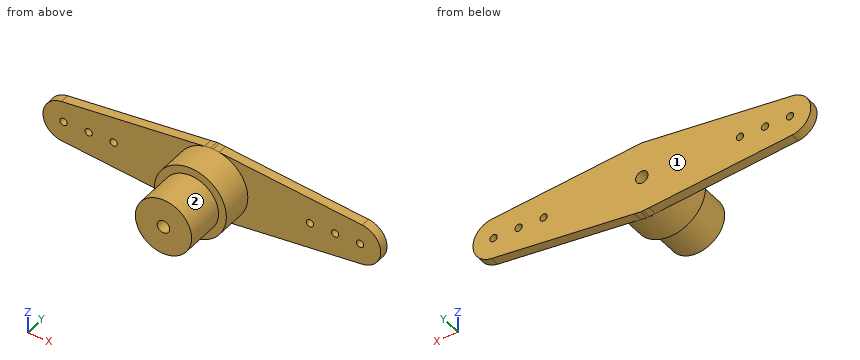
```python
from build123d import *

# Parameters (mm, degrees)
SKETCH1_R           = 2.875
BOSS_EXTRUDE1_DEPTH = 2.55
SKETCH1_4_R         = 0.291434634
BOSS_EXTRUDE2_DEPTH = 0.75
SKETCH2_R           = 2.25
BOSS_EXTRUDE3_DEPTH = 3.2
SKETCH3_R           = 0.5
CUT_EXTRUDE1_DEPTH  = 7.5
FILLET1_R           = 1


with BuildPart() as part:
    # Sketch1 → Boss-Extrude1 (new body)
    with BuildSketch(Plane(origin=(0, 0, 0), x_dir=(1, 0, 0), z_dir=(0, 1, 0))):
        Circle(SKETCH1_R)
    extrude(amount=-BOSS_EXTRUDE1_DEPTH)

    # Sketch1_4 → Boss-Extrude2 (add)
    with BuildSketch(Plane(origin=(0, 0, 0), x_dir=(1, 0, 0), z_dir=(0, 1, 0))):
        with BuildLine():
            Line((-0.584049273, 2.815050878), (-12.018477316, 1.641376067))
            ThreePointArc((-12.018477316, 1.641376067), (-13.5, 0), (-12.018477316, -1.641376067))
            Line((-12.018477316, -1.641376067), (-0.584049273, -2.815050878))
            ThreePointArc((-0.584049273, -2.815050878), (-2.875, 0), (-0.584049273, 2.815050878))
        make_face()
        with Locations((-11.85, 0)):
            Circle(SKETCH1_4_R, mode=Mode.SUBTRACT)
        with Locations((-9.85, 0)):
            Circle(SKETCH1_4_R, mode=Mode.SUBTRACT)
        with Locations((-7.85, 0)):
            Circle(SKETCH1_4_R, mode=Mode.SUBTRACT)
        with BuildLine():
            Line((12.018477316, 1.641376067), (0.584049273, 2.815050878))
            ThreePointArc((0.584049273, 2.815050878), (2.229884152, 1.81472909), (2.875, 0))
            ThreePointArc((2.875, 0), (2.229884152, -1.81472909), (0.584049273, -2.815050878))
            Line((0.584049273, -2.815050878), (12.018477316, -1.641376067))
            ThreePointArc((12.018477316, -1.641376067), (13.5, 0), (12.018477316, 1.641376067))
        make_face()
        with Locations((7.85, 0)):
            Circle(SKETCH1_4_R, mode=Mode.SUBTRACT)
        with Locations((9.85, 0)):
            Circle(SKETCH1_4_R, mode=Mode.SUBTRACT)
        with Locations((11.85, 0)):
            Circle(SKETCH1_4_R, mode=Mode.SUBTRACT)
        with BuildLine():
            Line((0, 2.875), (-0.584049273, 2.815050878))
            ThreePointArc((-0.584049273, 2.815050878), (-2.875, 0), (-0.584049273, -2.815050878))
            Line((-0.584049273, -2.815050878), (0, -2.875))
            Line((0, -2.875), (0.584049273, -2.815050878))
            ThreePointArc((0.584049273, -2.815050878), (2.229884152, -1.81472909), (2.875, 0))
            ThreePointArc((2.875, 0), (2.229884152, 1.81472909), (0.584049273, 2.815050878))
            Line((0.584049273, 2.815050878), (0, 2.875))
        make_face()
    extrude(amount=BOSS_EXTRUDE2_DEPTH)

    # Sketch2 → Boss-Extrude3 (add)
    with BuildSketch(Plane.XZ.offset(2.55)):
        Circle(SKETCH2_R)
    extrude(amount=BOSS_EXTRUDE3_DEPTH)

    # Sketch3 → Cut-Extrude1 (cut, through all)
    with BuildSketch(Plane.XZ.offset(5.75)):
        Circle(SKETCH3_R)
    extrude(amount=-CUT_EXTRUDE1_DEPTH, mode=Mode.SUBTRACT)

    # Fillet1
    fillet1_edges = [part.edges().sort_by_distance(p)[0] for p in [
        (0, 0.375, -2.875),
        (0, 0.375, 2.875),
    ]]
    fillet(fillet1_edges, radius=FILLET1_R)


solid = part.part
```
Design review of the part built by this model. Coordinates are the model's own, in mm. Face numbers are marked on the shaded views. A direction names the side the tool comes from. Coordinates: 2 decimals unless noted, no trailing zeros. Order: outer loops, then holes, each group sorted by start corner. A loop starts at its lowest first (then second) coordinate and runs counter-clockwise, first axis right, second up. Notation, with made-up numbers: M 47.25,44 L 59.25,44 A18 cw 59.25,72 Z; hole C 47,87 d1. An arc over 180 degrees is marked long. Answer as a JSON object with one key per item and string values. Group by question number.
1) For pin 1 (1.7 mm diameter, centred on x = 9.5, z = 1, fed in from -Y), flat-tipped, find the tip position at first contact; note if it passes through.
2) Tool access review of the marked faces 1 and 2: name each direction out of +Z, -Z, +X, -X, +Y, -Y from which nothing blocks a thin tool from reaching the whole face with its end or side.
3) Add section D-D, the plane y = -4.25. Write out the cut boundary in (x, z), then the cut area to 3 significant figures.
4) Add section B-B, the plane y = -1.5. Write out the cut boundary in (x, z) (3 decimals), then the cut area to 3 significant figures.
5) Add section A-A, the plane x = 7.85. Write out the cut boundary in (y, z), then the cut area to 3 significant figures.
6) Wall thickness on L1, parallel to Z at x = 0, y = -1 (3 decimals); L2, parallel to Y at x = -6.5, z = 0.7; L3, parallel to Z at x = -9.85, y = 0.5: over which ranges is each line inside the solid? List them lowest first.
7) Add section C-C, the plane x = -9.85. Write out the cut boundary in (y, z).
Computed values:
{
 "1": {"pin 1": "stops at y = 0"},
 "2": {"face 1": "+Z, -Z, +X, -X, +Y", "face 2": "-Y"},
 "3": {"outline": "C 0,0 d4.5; hole C 0,0 d1", "area": "15.1 mm^2"},
 "4": {"outline": "C 0,0 d5.75; hole C 0,0 d1", "area": "25.2 mm^2"},
 "5": {"outline": "M 0,-2.07 L 0.75,-2.07 L 0.75,-0.29 L 0,-0.29 Z; M 0,0.29 L 0.75,0.29 L 0.75,2.07 L 0,2.07 Z", "area": "2.67 mm^2"},
 "6": {"L1": "z = -2.875 to -0.5, 0.5 to 2.875", "L2": "y = 0 to 0.75", "L3": "z = -1.86 to -0.29, 0.29 to 1.86"},
 "7": {"outline": "M 0,-1.86 L 0.75,-1.86 L 0.75,-0.29 L 0,-0.29 Z; M 0,0.29 L 0.75,0.29 L 0.75,1.86 L 0,1.86 Z"}
}
